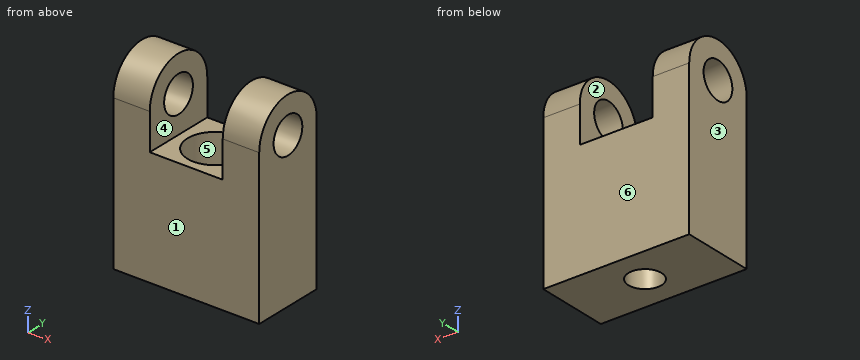
```python
from build123d import *

# Parameters (mm, degrees)
F1_DEPTH = 12.7
F2_R     = 1.5875
F3_DEPTH = 25.4
F5_DEPTH = 25.4
F7_DEPTH = 25.4
F8_R     = 2.3876
F9_DEPTH = 5.08


with BuildPart() as f1:
    # F0 (on Right) → F1 (new body)
    with BuildSketch(Plane.YZ):
        with BuildLine():
            Line((-3.175, 0), (0, 0))
            Line((0, 0), (3.175, 0))
            Line((3.175, 0), (3.175, 13.335))
            ThreePointArc((3.175, 13.335), (0, 16.51), (-3.175, 13.335))
            Line((-3.175, 13.335), (-3.175, 0))
        make_face()
    extrude(amount=F1_DEPTH)

    # F2 (on face) → F3 (cut)
    with BuildSketch(Plane.YZ.offset(12.7)):
        with Locations((0, 13.335)):
            Circle(F2_R)
    extrude(amount=-F3_DEPTH, mode=Mode.SUBTRACT)

    # F4 (on face) → F5 (cut)
    with BuildSketch(Plane.XZ.offset(3.175)):
        Polygon((3.175, 10.16), (6.35, 10.16), (9.525, 10.16), (9.525, 19.146023), (3.175, 19.146023), align=None)
    extrude(amount=-F5_DEPTH, mode=Mode.SUBTRACT)

    # F6 (on face) → F7 (cut)
    with BuildSketch(Plane.XY.offset(10.16)):
        with BuildLine():
            ThreePointArc((7.7851, 0), (6.35, 1.4351), (4.9149, 0))
            Line((4.9149, 0), (7.7851, 0))
        make_face()
        with BuildLine():
            Line((7.7851, 0), (4.9149, 0))
            ThreePointArc((4.9149, 0), (6.35, -1.4351), (7.7851, 0))
        make_face()
    extrude(amount=-F7_DEPTH, mode=Mode.SUBTRACT)

    # F8 (on face) → F9 (cut)
    with BuildSketch(Plane.XY.offset(10.16)):
        with Locations((6.35, 0)):
            Circle(F8_R)
    extrude(amount=-F9_DEPTH, mode=Mode.SUBTRACT)


solid = f1.part
```
The listing builds one solid part. Answer for the finished solid, in the listing's coordinates (mm). Face numbers are marked on the shaded views. A direction names the side the tool comes from. Round coordinates to 2 decimals unless told otherwise and drop trailing zeros. Loops run counter-clockwise (first coordinate to the right, second up) from the corner with the lowest first, then second, coordinate; pieces in that order, holes last.
Q1. Find the intervals of material crossed by line 1 (X direction, y = -0.5, z = 11.75) (3 decimals); line 2 (Z direction, x = 10.35, y = 0); line 3 (X direction, y = 0, z = 1.65), in increasing order.
Q2. Section B-B, the plane y = 0 is taken. Determine the outline of the cut face in (x, z) (1 decimal).
Q3. Section C-C, the plane z = 12.75 is taken. Determine the outline of the cut face in (x, y) (3 decimals), then the cut area to 3 significant figures.
Q4. Given pin 1 Ø3 at (x, y) = (6.5, -0.5) entering from +Z; pin 2 Ø1.9 at (y, z) = (-1, 13.5) entering from +X; pin 3 Ø2 at (x, y) = (4, -1) entering from +Z, each flat-ended and moving along its own axis, determine where each tip first touches the part or whether it passes through.
Q5. For a pull along X with two mould halves and no side action, classify the marked faces 1, 2 and 3 as released by +X, released by -X, zero draft, split by the parting line, or undercut.
Q6. Which of the six approach directions +Z, -Z, +X, -X, +Y, -Y give full straight-line access (tool end or side, diameter ignored) to the marked faces 4, 5 and 6?
Q7. Section A-A, the plane x = 6.35 is taken. Determine the outline of the cut face in (y, z) (3 decimals).
Completed:
1. line 1: x = 0 to 3.175, 9.525 to 12.7
1. line 2: z = 0 to 11.75, 14.92 to 16.51
1. line 3: x = 0 to 4.91, 7.79 to 12.7
2. outline: (0, 0) - (4.9, 0) - (4.9, 5.1) - (4, 5.1) - (4, 10.2) - (3.2, 10.2) - (3.2, 11.7) - (0, 11.7) - close; (0, 14.9) - (3.2, 14.9) - (3.2, 16.5) - (0, 16.5) - close; (7.8, 0) - (12.7, 0) - (12.7, 11.7) - (9.5, 11.7) - (9.5, 10.2) - (8.7, 10.2) - (8.7, 5.1) - (7.8, 5.1) - close; (9.5, 14.9) - (12.7, 14.9) - (12.7, 16.5) - (9.5, 16.5) - close
3. outline: (0, -3.175) - (3.175, -3.175) - (3.175, -1.476) - (0, -1.476) - close; (0, 1.476) - (3.175, 1.476) - (3.175, 3.175) - (0, 3.175) - close; (9.525, -3.175) - (12.7, -3.175) - (12.7, -1.476) - (9.525, -1.476) - close; (9.525, 1.476) - (12.7, 1.476) - (12.7, 3.175) - (9.525, 3.175) - close
3. area: 21.6 mm2
4. pin 1: stops at z = 5.08
4. pin 2: stops at x = 12.7
4. pin 3: stops at z = 16.48
5. face 1: zero draft
5. face 2: undercut
5. face 3: released by -X
6. face 4: +Z, +Y, -Y
6. face 5: +Z
6. face 6: +Z, -Z, +X, -X, +Y
7. outline: (-3.175, 0) - (-1.435, 0) - (-1.435, 5.08) - (-2.388, 5.08) - (-2.388, 10.16) - (-3.175, 10.16) - close; (1.435, 0) - (3.175, 0) - (3.175, 10.16) - (2.388, 10.16) - (2.388, 5.08) - (1.435, 5.08) - close
